from build123d import *

# Parameters (mm, degrees)
SKETCH1_R           = 23
BOSS_EXTRUDE1_DEPTH = 50
SKETCH2_R           = 8
BOSS_EXTRUDE2_DEPTH = 1
SKETCH5_R           = 1.5
CUT_EXTRUDE2_DEPTH  = 10
SKETCH6_R           = 1.5
CUT_EXTRUDE3_DEPTH  = 5
CIRPATTERN1_COUNT   = 4
CIRPATTERN2_COUNT   = 4
SKETCH7_R           = 5
BOSS_EXTRUDE3_DEPTH = 5
SKETCH8_R           = 2.425
BOSS_EXTRUDE4_DEPTH = 5


with BuildPart() as part:
    # Sketch1 → Boss-Extrude1 (new body)
    with BuildSketch(Plane.XY):
        Circle(SKETCH1_R)
    extrude(amount=-BOSS_EXTRUDE1_DEPTH)

    # Sketch2 → Boss-Extrude2 (add)
    with BuildSketch(Plane.XY):
        Circle(SKETCH2_R)
    extrude(amount=BOSS_EXTRUDE2_DEPTH)

    # Sketch5 → Cut-Extrude2 (cut)
    with BuildSketch(Plane(origin=(0, 0, -50), x_dir=(-1, 0, 0), z_dir=(0, 0, -1))):
        with Locations((-12.5, 0)):
            Circle(SKETCH5_R)
    cut_extrude2 = extrude(amount=-CUT_EXTRUDE2_DEPTH, mode=Mode.SUBTRACT)

    # Sketch6 → Cut-Extrude3 (cut)
    with BuildSketch(Plane.XY):
        with Locations((0, 14)):
            Circle(SKETCH6_R)
    cut_extrude3 = extrude(amount=-CUT_EXTRUDE3_DEPTH, mode=Mode.SUBTRACT)

    # CirPattern1: Cut-Extrude3 ×4 about axis
    cirpattern1_axis = Axis((0, 0, 0), (0, 0, 1))
    for i in range(1, CIRPATTERN1_COUNT):
        add(cut_extrude3.rotate(cirpattern1_axis, i * 360 / CIRPATTERN1_COUNT), mode=Mode.SUBTRACT)

    # CirPattern2: Cut-Extrude2 ×4 about axis
    cirpattern2_axis = Axis((0, 0, 0), (0, 0, 1))
    for i in range(1, CIRPATTERN2_COUNT):
        add(cut_extrude2.rotate(cirpattern2_axis, i * 360 / CIRPATTERN2_COUNT), mode=Mode.SUBTRACT)

    # Sketch7 → Boss-Extrude3 (add)
    with BuildSketch(Plane(origin=(0, 0, -50), x_dir=(-1, 0, 0), z_dir=(0, 0, -1))):
        Circle(SKETCH7_R)
    extrude(amount=BOSS_EXTRUDE3_DEPTH)

    # Sketch8 → Boss-Extrude4 (add)
    with BuildSketch(Plane(origin=(0, 0, -55), x_dir=(-1, 0, 0), z_dir=(0, 0, -1))):
        Circle(SKETCH8_R)
    extrude(amount=BOSS_EXTRUDE4_DEPTH)


solid = part.part
Read the model definition and answer for the solid it produces. Units are mm, in the model's axes. A direction names the side the tool comes from. Round coordinates to 2 decimals unless told otherwise and drop trailing zeros. Write each loop counter-clockwise with the first axis right and the second up, starting at its lowest first coordinate (ties: lowest second). Pieces come first, ordered by that corner, then holes.
1. Straight lines are drawn through the part: L1, parallel to Y at x = 0, z = -3; L2, parallel to Z at x = 20.5, y = -10; L3, parallel to Z at x = -0.5, y = -4. For each, find the intervals that lie inside material, in ascending order.
2. The part is cut by section B-B, the plane z = -42. Determine the outline of the cut face in (x, y), then the cut area to 3 significant figures.
3. Which of the six approach directions +Z, -Z, +X, -X, +Y, -Y give full straight-line access (tool end or side, diameter ignored) to faces 1 (the face through (0, 0, -60)), 2 (the face through (12.536, 0.325, -2.465)), 3 (the face through (13, 0, -40))?
4. The part is cut by section D-D, the plane z = -20. Determine the outline of the cut face in (x, y).
5. Determine the mould class of faces 4 (the face through (0, 14, -5)), 5 (the face through (10, 0, 0)), 6 (the face through (-1.73, -7.81, 0.49)) for opening direction Y: pulls with the +Y half, pulls with the -Y half, needs draft (parallel to the pull), parting line crosses it, or undercut.
6. Given pin 1 Ø1.5 at (x, y) = (0, -12.5) entering from -Z; pin 2 Ø3.5 at (x, y) = (12.5, 0.5) entering from -Z; pin 3 Ø4 at (x, y) = (0, -14) entering from +Z; pin 4 Ø14 at (x, y) = (-10, 2.5) entering from +Z, each flat-ended and moving along its own axis, determine where each tip first touches the part or whether it passes through.
Values:
1. L1: y = -23 to -15.5, -12.5 to 12.5, 15.5 to 23
1. L2: z = -50 to 0
1. L3: z = -55 to 1
2. outline: circle Ø46 at (0, 0); hole circle Ø3 at (-12.5, 0); hole circle Ø3 at (0, -12.5); hole circle Ø3 at (0, 12.5); hole circle Ø3 at (12.5, 0)
2. area: 1,630 mm2
3. face 1: -Z, +X, -X, +Y, -Y
3. face 2: +Z
3. face 3: -Z
4. outline: circle Ø46 at (0, 0)
5. face 4: undercut
5. face 5: needs draft
5. face 6: parting line crosses it
6. pin 1: stops at z = -40
6. pin 2: stops at z = -50
6. pin 3: stops at z = 0
6. pin 4: stops at z = 1
